Part model, mm, in its own coordinate system. A direction names the side the tool comes from. Round coordinates to 2 decimals unless told otherwise and drop trailing zeros. Loops run counter-clockwise (first coordinate to the right, second up) from the corner with the lowest first, then second, coordinate; pieces in that order, holes last. Notation, with made-up numbers: (86, 51) -> (125, 51) arc R18 cw to (125, 79) -> close; hole circle Ø4 at (86, -14). An arc over 180 degrees is marked (long way). Answer as CSV lines item,"result".
Autodesk Inventor part; units mm, degrees
ref_plane "YZ Plane" through (0, 0, 0) normal (1, 0, 0) x (0, 1, 0)
ref_plane "XZ Plane" through (0, 0, 0) normal (0, 1, 0) x (-1, 0, 0)
ref_plane "XY Plane" through (0, 0, 0) normal (0, 0, 1) x (1, 0, 0)
sketch "スケッチ1" plane through (0, 0, 0) normal (1, 0, 0) x (0, 1, 0)
  line L0 (35, -42.2311) -> (-5, -42.2311)
  line L1 (-5, -42.2311) -> (-5, -102.2311)
  line L2 (-5, -102.2311) -> (35, -102.2311)
  line L3 (35, -102.2311) -> (35, -42.2311)
  line L4 (30, 7.7689) -> (0, 7.7689)
  line L5 (0, 7.7689) -> (0, -42.2311)
  line L6 (0, -42.2311) -> (30, -42.2311)
  line L7 (30, -42.2311) -> (30, 7.7689)
  dimension "d1" = 40
  dimension "d2" = 60
  dimension "d68" = 30
  dimension "d69" = 50
  dimension "d70" = 0
  dimension "d71" = 5
extrude "押し出し1" add sketch "スケッチ1" along normal blind 3
sketch "スケッチ4" plane through (3, 0, 0) normal (1, 0, 0) x (0, 0, -1)
  line L0 (56.2311, 30) -> (97.2311, 30)
  line L1 (97.2311, 30) -> (97.2311, 0)
  line L2 (97.2311, 0) -> (56.2311, 0)
  line L3 (56.2311, 0) -> (56.2311, 30)
  line L4 (102.2311, 35) -> (42.2311, 35)
  line L5 (102.2311, -5) -> (102.2311, 35)
  point P0 (0, 0)
  dimension "d29" = 41
  dimension "d30" = 30
  dimension "d31" = 5
  dimension "d32" = 5
hole "穴2" at (3, 30, -56.2311) at (3, 0, -56.2311) at (3, 0, -97.2311) at (3, 30, -97.2311) direction (-1, 0, 0) diameter 3.2 end through all
sketch "スケッチ7" plane through (3, 0, 0) normal (1, 0, 0) x (0, 0, -1)
  line L0 (102.2311, -5) -> (102.2311, 35)
  line L1 (102.2311, 15) -> (-7.7689, 15)
  line L2 (-7.7689, 30) -> (-7.7689, 0)
  point P0 (0, 0)
  point P1 (-0.7689, 15)
  point P2 (29.2311, 15)
  dimension "d72" = 7
  dimension "d73" = 30
hole "穴5" at (3, 15, 0.7689) at (3, 15, -29.2311) direction (-1, 0, 0) diameter 4.2 end through all
properties part number "link4_plate1" material "アルミニウム 6061"
Q1. Saw through at A-A, the plane y = 15. Write the cut outline in (x, z), then the cut area to 3 significant figures.
Geometry results:
outline,"(0, -102.23) -> (3, -102.23) -> (3, -31.33) -> (0, -31.33) -> close; (0, -27.13) -> (3, -27.13) -> (3, -1.33) -> (0, -1.33) -> close; (0, 2.87) -> (3, 2.87) -> (3, 7.77) -> (0, 7.77) -> close"
area,"305 mm2"
Q2. Saw through at C-C, the plane z = -11. Write the cut outline in (x, y), then the cut area to 3 significant figures.
Geometry results:
outline,"(0, 0) -> (3, 0) -> (3, 30) -> (0, 30) -> close"
area,"90.0 mm2"
Q3. Which spindle directions (+Z, -Z, +X, -X, +Y, -Y) get a long thin tool onto all of the face, cutting with end or side? Do faces 1 (the face through (1, 33, -42.231)), 2 (the face through (3, 15, -46)), 3 (the face through (1, 0, -17)). Say none if no direction does.
Geometry results:
face 1,"+Z, +X, -X, +Y"
face 2,"+Z, -Z, +X, +Y, -Y"
face 3,"+Z, +X, -X, -Y"
Q4. Drill centre lines: line 1 along Z through (x, y) = (1, 15); line 2 along Y through (x, z) = (1.2, -8); line 3 along Y through (x, z) = (0.7, 2). Where is each one in solid material? Low to high.
Geometry results:
line 1,"-102.23 to -31.33, -27.13 to -1.33, 2.87 to 7.77"
line 2,"0 to 30"
line 3,"0 to 13.3, 16.7 to 30"
Q5. Drop flat-ended pins along their axis: P1, Ø0.9, axis at x = 2, y = -3.5, coming from the +Z side; P2, Ø2.5, axis at y = 30, z = -97.23, coming from the -X side; P3, Ø4, axis at y = 1, z = -56.5, coming from the -X side; P4, Ø1.5, axis at x = 2, z = -27, coming from the -Y side. Give the stop position or say it passes through.
Geometry results:
P1,"z = -42.23"
P2,"through"
P3,"x = 0"
P4,"y = 0"
Q6. Two-plate mould, pull along Z, no slides. Class faces 4 (the face through (1, 15, 7.769)), 5 (the face through (1, 30, -18)), 6 (the face through (1.48, 28.65, -57.09)): pulls with the +Z half, pulls with the -Z half, needs draft (parallel to the pull), parting line crosses it, or undercut.
Geometry results:
face 4,"pulls with the +Z half"
face 5,"needs draft"
face 6,"undercut"
Q7. Saw through at B-B, the plane x = 2.1. Write the cut outline in (y, z).
Geometry results:
outline,"(-5, -102.23) -> (35, -102.23) -> (35, -42.23) -> (30, -42.23) -> (30, 7.77) -> (0, 7.77) -> (0, -42.23) -> (-5, -42.23) -> close; hole circle Ø3.2 at (0, -97.23); hole circle Ø3.2 at (0, -56.23); hole circle Ø4.2 at (15, -29.23); hole circle Ø4.2 at (15, 0.77); hole circle Ø3.2 at (30, -97.23); hole circle Ø3.2 at (30, -56.23)"
